Verification items for the finished model (mm, model axes). Coordinates: 2 decimals unless noted, no trailing zeros. Order: outer loops, then holes, each group sorted by start corner. A loop starts at its lowest first (then second) coordinate and runs counter-clockwise, first axis right, second up. Notation, with made-up numbers: (-36, 45) -> (-28, 45) arc R10 ccw to (-28, 62) -> close; hole circle Ø2 at (-37, 39). An arc over 180 degrees is marked (long way). Write each question's results on one line, items separated by ' | '. Start each with the question number.
(1) Cross-section at A-A on x = -77.5. Enter the section's corners in (y, z), and give its area (3 significant figures).
(2) Cross-section at B-B on y = 27.75. Enter the section's corners in (x, z).
(3) Cross-section at C-C on z = 0.95. Enter the section's corners in (x, y), and give its area (3 significant figures).
(4) Thickness scan on probe 1 along X at (y, z) = (26, 2.65); probe 2 along X at (y, z) = (25.75, 1.5); probe 3 along Y at (x, z) = (-78, 2.15). Record the ranges inside material, lowest first. Write a range as [from, to].
(5) Cross-section at D-D on x = -50. Enter the section's corners in (y, z).
(6) Draft check along X on faces 1 (the cylindrical face through (-53.29, 24.8, 1.48)), 2 (the cylindrical face through (-83.014, 25.91, 1.479)), 3 (the flat face through (-65, 21.02, 1)). Enter one of: +X half, -X half, draft (parallel to the pull), parting line (faces both ways), or undercut.
```python
from build123d import *
from build123d.topology import SkipClean

# Parameters (mm, degrees)
SKETCH1_R           = 1.5
SKETCH1_R_2         = 1.25
BOSS_EXTRUDE1_DEPTH = 3
SKETCH5_R           = 2.1
CUT_EXTRUDE2_DEPTH  = 10
BOSS_EXTRUDE2_DEPTH = 3


with BuildPart() as part:
    # Sketch1 → Boss-Extrude1 (new body)
    with BuildSketch(Plane.XY):
        with BuildLine():
            Line((-78.015219505, 31.020337279), (-53.015219505, 31.020337279))
            ThreePointArc((-53.015219505, 31.020337279), (-48.015219505, 26.020337279), (-53.015219505, 21.020337279))
            Line((-53.015219505, 21.020337279), (-78.015219505, 21.020337279))
            ThreePointArc((-78.015219505, 21.020337279), (-83.015219505, 26.020337279), (-78.015219505, 31.020337279))
        make_face()
        with Locations((-63.015219505, 26.020337279)):
            Circle(SKETCH1_R, mode=Mode.SUBTRACT)
        with Locations((-53.015219505, 26.020337279)):
            Circle(SKETCH1_R_2, mode=Mode.SUBTRACT)
        with Locations((-78.015219505, 26.020337279)):
            Circle(SKETCH1_R_2, mode=Mode.SUBTRACT)
    extrude(amount=BOSS_EXTRUDE1_DEPTH)

    # Sketch5 → Cut-Extrude2 (cut)
    with BuildSketch(Plane.XY.offset(3)):
        with Locations((-66.015219505, 26.020337279)):
            Circle(SKETCH5_R)
    extrude(amount=-CUT_EXTRUDE2_DEPTH, mode=Mode.SUBTRACT)

    # Sketch6 → Boss-Extrude2 (add)
    with SkipClean():  # the faces are left unmerged after this step: merging them gives an invalid solid
        with BuildSketch(Plane.XY.offset(3)):
            with BuildLine():
                ThreePointArc((-64.155219505, 25.045452671), (-61.515219505, 26.020337279), (-64.155219505, 26.995221888))
                ThreePointArc((-64.155219505, 26.995221888), (-63.915219505, 26.020337279), (-64.155219505, 25.045452671))
            make_face()
        extrude(amount=-BOSS_EXTRUDE2_DEPTH)


solid = part.part
```
Results are:
1) outline: (21.02, 0) -> (24.88, 0) -> (24.88, 3) -> (21.02, 3) -> close; (27.16, 0) -> (31.02, 0) -> (31.02, 3) -> (27.16, 3) -> close | area: 23.2 mm2
2) outline: (-82.71, 0) -> (-67.21, 0) -> (-67.21, 3) -> (-82.71, 3) -> close; (-64.82, 0) -> (-48.32, 0) -> (-48.32, 3) -> (-64.82, 3) -> close
3) outline: (-78.02, 21.02) -> (-53.02, 21.02) arc R5 ccw to (-53.02, 31.02) -> (-78.02, 31.02) arc R5 ccw to start; hole circle Ø2.5 at (-78.02, 26.02); hole circle Ø4.2 at (-66.02, 26.02); hole circle Ø2.5 at (-53.02, 26.02) | area: 305 mm2
4) probe 1: x = [-83.02, -79.27], [-76.77, -68.12], [-63.92, -54.27], [-51.77, -48.02] | probe 2: x = [-83.01, -79.24], [-76.79, -68.1], [-63.93, -54.24], [-51.79, -48.02] | probe 3: y = [21.02, 24.77], [27.27, 31.02]
5) outline: (22.03, 0) -> (30.01, 0) -> (30.01, 3) -> (22.03, 3) -> close
6) face 1: undercut | face 2: -X half | face 3: draft
